```python
from build123d import *

# Parameters (mm, degrees)
CUT_EXTRUDE1_DEPTH = 65
SKETCH4_W          = 2.495898364
SKETCH4_H          = 1.5
FILLET1_R          = 1.5
FILLET2_R          = 1.5
FILLET3_R          = 1.5


with BuildPart() as part:
    # Sketch1 → Revolve1 (revolve)
    with BuildSketch(Plane.XY):
        with BuildLine():
            Line((0, 74.75), (0, 73.175))
            ThreePointArc((0, 73.175), (73.175, 0), (0, -73.175))
            Line((0, -73.175), (0, -74.75))
            ThreePointArc((0, -74.75), (74.75, 0), (0, 74.75))
        make_face()
    revolve(axis=Axis((0, 74.75, 0), (0, -1, 0)))

    # Sketch3 → Cut-Extrude1 (cut, symmetric)
    with BuildSketch(Plane.XY):
        Polygon((45.425, -57.368545389), (-45.425, -57.368545389), (-47.920898364, -57.368545389), (-47.920898364, -74.75), (47.920898364, -74.75), (47.920898364, -57.368545389), align=None)
    extrude(amount=CUT_EXTRUDE1_DEPTH, both=True, mode=Mode.SUBTRACT)

    # Sketch4 → Revolve2 (revolve)
    with BuildSketch(Plane.XY, mode=Mode.PRIVATE) as revolve2_sk:
        with Locations((46.672949182, -58.118545389)):
            Rectangle(SKETCH4_W, SKETCH4_H)
    revolve(revolve2_sk.sketch.rotate(Axis((0, -73.175, 0), (0, -1, 0)), 180), axis=Axis((0, -73.175, 0), (0, -1, 0)))

    # Fillet1
    fillet1_edges = [part.edges().sort_by_distance(p)[0] for p in [
        (47.920898364, -58.868545389, 0),
    ]]
    fillet(fillet1_edges, radius=FILLET1_R - 0.0001)  # a hair under: the kernel refuses the full size

    # Fillet2
    fillet2_edges = [part.edges().sort_by_distance(p)[0] for p in [
        (0, -57.368545389, -47.920898364),
    ]]
    fillet(fillet2_edges, radius=FILLET2_R)

    # Fillet3
    fillet3_edges = [part.edges().sort_by_distance(p)[0] for p in [
        (0, -57.368545389, -45.425),
    ]]
    fillet(fillet3_edges, radius=FILLET3_R)


solid = part.part
```
Could you check a few things on this model? Use its own coordinates, in mm. Coordinates: 2 decimals unless noted, no trailing zeros. Write each loop counter-clockwise with the first axis right and the second up, starting at its lowest first coordinate (ties: lowest second). Pieces come first, ordered by that corner, then holes. Notation, with made-up numbers: (34.25, 87.25) -> (51.25, 87.25) arc R14 ccw to (51.25, 109.25) -> close; hole circle Ø8 at (13, 2.25). An arc over 180 degrees is marked (long way). Write item = value, one per line. Start each with the question number.
(1) I need wall thicknesses on line 1 (Y direction, x = 55.5, z = 15); line 2 (X direction, y = 36, z = -0.5); line 3 (Z direction, x = 0, y = -58). Which ranges of each line are inside material? Lowest first, please. Write a range as [from, to].
(2) We'd pull the mould along Z, two halves only. Please class faces 1 (the face through (-43.33, -58.47, -13.64)), 2 (the face through (31, -58.869, 34)): released by +Z, released by -Z, zero draft, split by the parting line, or undercut.
(3) Will these pins go through, and if not, where does the flat tip stop? pin 1 (1.5 mm diameter, centred on x = -44.5, y = -16, fed in from +Z); pin 2 (5 mm diameter, centred on y = -32.5, z = 45, fed in from +X); pin 3 (1.5 mm diameter, centred on y = -26, z = 11, fed in from +X).
(4) I want a section at B-B (z = -53). Please give me the cut outline in (x, y), plus the area to 3 significant figures.
Result set:
q1.line_1 = [-47.77, -45.27], [45.27, 47.77]
q1.line_2 = [-65.51, -63.71], [63.71, 65.51]
q1.line_3 = [-47.78, -45.43], [45.43, 47.78]
q2.face_1 = undercut
q2.face_2 = zero draft
q3.pin_1 = 58.5
q3.pin_2 = 52.7
q3.pin_3 = 69.52
q4.outline = circle Ø105.42 at (0, 0); hole circle Ø100.91 at (0, 0)
q4.area = 732 mm2
